```python
from build123d import *

# Parameters (mm, degrees)
F1_DEPTH = 25.4
F2_W     = 43.18
F2_H     = 17.78
F3_DEPTH = 50.801
F4_W     = 12.7
F4_H     = 8.7366292986
F5_DEPTH = 7.621
F6_R     = 19.05
F7_DEPTH = 7.621


with BuildPart() as f1:
    # F0 (on Top) → F1 (new body)
    with BuildSketch(Plane.XY):
        with BuildLine():
            Line((25.4, 25.4), (-25.4, 25.4))
            Line((-25.4, 25.4), (-25.4, -25.4))
            ThreePointArc((-25.4, -25.4), (0, -50.8), (25.4, -25.4))
            Line((25.4, -25.4), (25.4, 25.4))
        make_face()
    extrude(amount=F1_DEPTH)

    # F2 (on face) → F3 (cut, through all)
    with BuildSketch(Plane.YZ.offset(25.4)):
        with Locations((-3.81, 16.51)):
            Rectangle(F2_W, F2_H)
        Polygon((17.78, 33.02), (-60.672249645, 33.02), (-60.672249645, 7.62), (-25.4, 7.62), (-25.4, 25.4), (17.78, 25.4), align=None)
    extrude(amount=-F3_DEPTH, mode=Mode.SUBTRACT)

    # F4 (on face) → F5 (cut, through all)
    with BuildSketch(Plane.XZ.offset(-17.78)):
        with Locations((-19.05, 21.0316853507)):
            Rectangle(F4_W, F4_H)
    extrude(amount=-F5_DEPTH, mode=Mode.SUBTRACT)

    # F6 (on face) → F7 (cut, through all)
    with BuildSketch(Plane.XY.offset(7.62)):
        with Locations((0, -25.4)):
            Circle(F6_R)
    extrude(amount=-F7_DEPTH, mode=Mode.SUBTRACT)


solid = f1.part
```
Geometry: final body of the model. Coordinates: model frame, mm. A direction names the side the tool comes from. Round coordinates to 2 decimals unless told otherwise and drop trailing zeros. Write each loop counter-clockwise with the first axis right and the second up, starting at its lowest first coordinate (ties: lowest second). Pieces come first, ordered by that corner, then holes. Notation, with made-up numbers: (57.5, -20) -> (84.5, -20) arc R35 ccw to (84.5, 19) -> close; hole circle Ø5 at (33, -31.75). An arc over 180 degrees is marked (long way). Use CSV: the item, a comma, the result in double quotes. Start each with the question number.
Q1. Reachability of faces 4 (the face through (25.4, 5, 7)), 5 (the face through (0, 17.78, 16)), 6 (the face through (-12.7, 22, 21)) from +Z, -Z, +X, -X, +Y, -Y: full face, straight path, thin tool, end or side. Return the list, or none.
Q2. Section B-B (y = -10.5). Return loops of the section in (x, z).
Q3. Pull-direction query (Y, two-part tool) for faces 1 (the face through (-0.559, -50.794, 3.757)), 2 (the face through (6, 22, 25.4)), 3 (the face through (-2.48, -6.512, 3.863)); classes: pulls with the +Y half, pulls with the -Y half, needs draft (parallel to the pull), parting line crosses it, or undercut.
Q4. First-contact query: pin 1 Ø2 at (x, z) = (13, 7.5) entering from -Y; pin 2 Ø9 at (x, z) = (5, 12.5) entering from -Y; pin 3 Ø8.5 at (y, z) = (20, 23) entering from -X; pin 4 Ø5 at (x, y) = (14, -6.5) entering from -Z. Flat tips, straight axial feed; report the tip coordinate or a pass-through.
Q5. Section C-C (x = -10.5). Return loops of the section in (y, z), plus the area to 3 significant figures.
Q6. Section A-A (x = 0). Return loops of the section in (y, z).
Q7. Line query: L1, parallel to Y at x = 0, z = 1.75; L2, parallel to Z at x = -9.5, y = 7; L3, parallel to Y at x = 2.5, z = 13.5. Output: solid intervals per line, ascending.
Q8. Section D-D (y = -37). Return loops of the section in (x, z).
Result sheet:
1,face 4,"+Z, -Z, +X, +Y, -Y"
1,face 5,"+Z, +X, -X, -Y"
1,face 6,"+Z, -X, +Y, -Y"
2,outline,"(-25.4, 0) -> (-11.87, 0) -> (-11.87, 7.62) -> (-25.4, 7.62) -> close; (11.87, 0) -> (25.4, 0) -> (25.4, 7.62) -> (11.87, 7.62) -> close"
3,face 1,"pulls with the -Y half"
3,face 2,"needs draft"
3,face 3,"undercut"
4,pin 1,"y = -47.79"
4,pin 2,"y = 17.78"
4,pin 3,"x = -12.7"
4,pin 4,"z = 0"
5,outline,"(-48.53, 0) -> (-41.3, 0) -> (-41.3, 7.62) -> (-48.53, 7.62) -> close; (-9.5, 0) -> (25.4, 0) -> (25.4, 25.4) -> (17.78, 25.4) -> (17.78, 7.62) -> (-9.5, 7.62) -> close"
5,area,"457 mm²"
6,outline,"(-50.8, 0) -> (-44.45, 0) -> (-44.45, 7.62) -> (-50.8, 7.62) -> close; (-6.35, 0) -> (25.4, 0) -> (25.4, 25.4) -> (17.78, 25.4) -> (17.78, 7.62) -> (-6.35, 7.62) -> close"
7,L1,"-50.8 to -44.45, -6.35 to 25.4"
7,L2,"0 to 7.62"
7,L3,"17.78 to 25.4"
8,outline,"(-22.6, 0) -> (-15.11, 0) -> (-15.11, 7.62) -> (-22.6, 7.62) -> close; (15.11, 0) -> (22.6, 0) -> (22.6, 7.62) -> (15.11, 7.62) -> close"
